The model under review builds one solid part; all positions refer to its coordinate system, in mm. Face numbers are marked on the shaded views. A direction names the side the tool comes from. Round coordinates to 2 decimals unless told otherwise and drop trailing zeros. Loops run counter-clockwise (first coordinate to the right, second up) from the corner with the lowest first, then second, coordinate; pieces in that order, holes last. Notation, with made-up numbers: M -16,83.25 L -3,83.25 A7 cw -3,92.25 Z; hole C 24,0 d4. An arc over 180 degrees is marked long. Use a Markdown table: item, result. Add a question column.
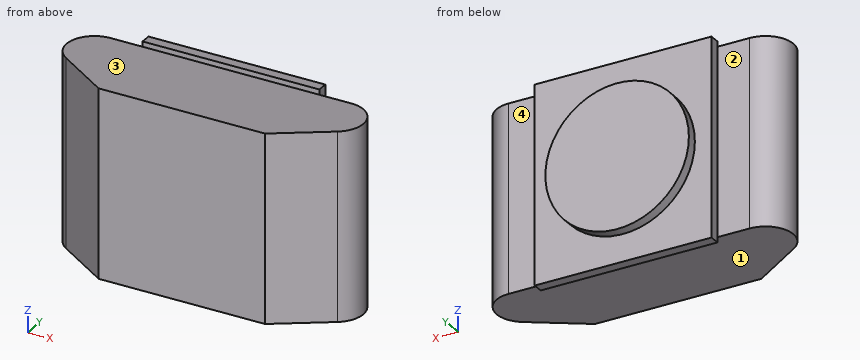
Autodesk Inventor part; units mm, degrees
ref_plane "YZ Plane" through (0, 0, 0) normal (1, 0, 0) x (0, 1, 0)
ref_plane "XZ Plane" through (0, 0, 0) normal (0, 1, 0) x (-1, 0, 0)
ref_plane "XY Plane" through (0, 0, 0) normal (0, 0, 1) x (1, 0, 0)
sketch "Sketch1" plane through (0, 0, 0) normal (0, 0, 1) x (1, 0, 0)
  line L0 (-142.5, 102) -> (142.5, 102) construction
  line L1 (142.5, 102) -> (142.5, 82) construction
  line L2 (142.5, 0) -> (-142.5, 0)
  line L3 (-142.5, 0) -> (-142.5, 82)
  line L4 (-142.5, 82) -> (142.5, 82)
  line L5 (142.5, 82) -> (142.5, 0)
  line L6 (80, 0) -> (142.5, 41)
  circle A0 centre (115.876, 55.376) radius 26.624
  line L7 (-142.5, 82) -> (-142.5, 102) construction
  line L8 (-80, 0) -> (-142.5, 41)
  circle A1 centre (-115.876, 55.376) radius 26.624
  point P0 (0, 0)
  point P1 (0, 0)
  point P2 (-130.4796, 33.1146)
  point P3 (130.4796, 33.1146)
  point P4 (115.876, 82)
  point P5 (-115.876, 82)
  dimension "d7" = 285
  dimension "d8" = 102
  dimension "d9" = 82
  dimension "d13" = 80
  dimension "d14" = 80
extrude "Extrusion1" add sketch "Sketch1" along normal mid plane 180 contours L2 L8 A1 L4 A0 L6 | A0 | A1
sketch "Sketch2" plane through (-115.876, 82, 90) normal (0, 1, 0) x (1, 0, 0)
  line L0 (30.876, -5) -> (200.876, -5)
  line L1 (200.876, -5) -> (200.876, 185)
  line L2 (200.876, 185) -> (30.876, 185)
  line L3 (30.876, 185) -> (30.876, -5)
  line L4 (30.876, -5) -> (200.876, 185) construction
  point P0 (115.876, 90)
  point P1 (115.876, 90)
  dimension "d17" = 190
  dimension "d18" = 170
extrude "Extrusion2" add sketch "Sketch2" along normal blind 10
sketch "Sketch3" plane through (0, 0, 0) normal (0, 1, 0) x (-1, 0, 0)
  circle A0 centre (0, 0) radius 69
  dimension "d21" = 138
extrude "Extrusion3" add sketch "Sketch3" along normal blind 102
properties part number "Roller platform"
(1) Consider section A-A, the plane x = 0. Give the boundary of the cut face in (y, z).
(2) Insertion check: pin 1 Ø1 at (y, z) = (80, 23.5) entering from +X; pin 2 Ø24.5 at (x, y) = (49.5, 37) entering from +Z; pin 3 Ø4 at (y, z) = (25, 51.5) entering from +X. Each pin has a flat end and moves straight along its axis. Give the tip position at first contact, or say it passes through.
(3) Consider section D-D, the plane z = -53. Give the boundary of the cut face in (x, y), then the cut area to 3 significant figures.
(4) For the marked faces 1, 2, 3 and 4, list the 3-axis set-ups (+Z, -Z, +X, -X, +Y, -Y) from which the entire face can be reached by the end or side of a thin tool; tool diameter is ignored.
(5) Consider section B-B, the plane z = -76. Give the boundary of the cut face in (x, y), then the cut area to 3 significant figures.
(6) Consider section C-C, the plane y = 28. Give the boundary of the cut face in (x, z).
(7) To check wall thickness, follow probe 1 along Z at (x, y) = (-101.5, 55.5); probe 2 along Y at (x, z) = (40.5, 79.5); probe 3 along X at (y, z) = (56.5, -79). State the ranges of each line that lie inside material, in increasing order.
Found:
| question | item | result |
|---|---|---|
| 1 | outline | M 0,-90 L 82,-90 L 82,-95 L 92,-95 L 92,-69 L 102,-69 L 102,69 L 92,69 L 92,95 L 82,95 L 82,90 L 0,90 Z |
| 2 | pin 1 | stops at x = 127.14 |
| 2 | pin 2 | stops at z = 90 |
| 2 | pin 3 | stops at x = 121.16 |
| 3 | outline | M -130.48,33.11 L -80,0 L 80,0 L 130.48,33.11 A26.62 ccw 115.88,82 L 85,82 L 85,92 L 44.18,92 L 44.18,102 L -44.18,102 L -44.18,92 L -85,92 L -85,82 L -115.88,82 A26.62 ccw Z |
| 3 | area | 23,000 mm^2 |
| 4 | face 1 | -Z, +X, -X, -Y |
| 4 | face 2 | +Z, -Z, -X, +Y |
| 4 | face 3 | +Z, +X, -X, -Y |
| 4 | face 4 | +Z, -Z, +X, +Y |
| 5 | outline | M -130.48,33.11 L -80,0 L 80,0 L 130.48,33.11 A26.62 ccw 115.88,82 L 85,82 L 85,92 L -85,92 L -85,82 L -115.88,82 A26.62 ccw Z |
| 5 | area | 22,100 mm^2 |
| 6 | outline | M -122.68,-90 L 122.68,-90 L 122.68,90 L -122.68,90 Z |
| 7 | probe 1 | z = -90 to 90 |
| 7 | probe 2 | y = 0 to 92 |
| 7 | probe 3 | x = -142.48 to 142.48 |
